Geometry: final body of the model. Coordinates: model frame, mm. Face numbers are marked on the shaded views. Coordinates: 2 decimals unless noted, no trailing zeros. Write each loop counter-clockwise with the first axis right and the second up, starting at its lowest first coordinate (ties: lowest second). Pieces come first, ordered by that corner, then holes.
from build123d import *

# Parameters (mm, degrees)
SKETCH1_W           = 150
SKETCH1_H           = 150
BOSS_EXTRUDE1_DEPTH = 19
SKETCH2_R           = 28
CUT_EXTRUDE1_DEPTH  = 3
SKETCH4_R           = 2.5
CUT_EXTRUDE2_DEPTH  = 6.35


with BuildPart() as part:
    # Sketch1 → Boss-Extrude1 (new body)
    with BuildSketch(Plane(origin=(0, 0, 0), x_dir=(1, 0, 0), z_dir=(0, 1, 0))):
        with Locations((75, 75)):
            Rectangle(SKETCH1_W, SKETCH1_H)
    extrude(amount=BOSS_EXTRUDE1_DEPTH)

    # Sketch2 → Cut-Extrude1 (cut)
    with BuildSketch(Plane(origin=(0, 19, 0), x_dir=(1, 0, 0), z_dir=(0, 1, 0))):
        with Locations((75, 75)):
            Circle(SKETCH2_R)
    extrude(amount=-CUT_EXTRUDE1_DEPTH, mode=Mode.SUBTRACT)

    # Sketch4 → Cut-Extrude2 (cut)
    with BuildSketch(Plane(origin=(0, 19, 0), x_dir=(1, 0, 0), z_dir=(0, 1, 0))):
        with Locations((10, 140)):
            Circle(SKETCH4_R)
        with Locations((140, 140)):
            Circle(SKETCH4_R)
        with Locations((140, 10)):
            Circle(SKETCH4_R)
        with Locations((10, 10)):
            Circle(SKETCH4_R)
    extrude(amount=-CUT_EXTRUDE2_DEPTH, mode=Mode.SUBTRACT)


solid = part.part
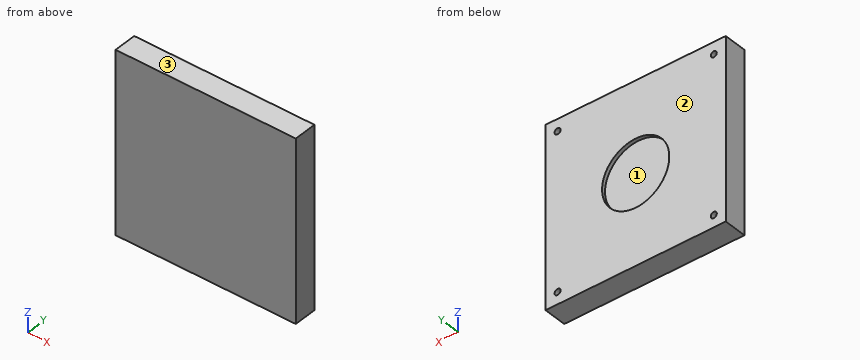
Item 1: Section D-D, the plane x = 10. Output: boundary loops of the cut face in (y, z).
Derived:
outline: (0, -150) - (19, -150) - (19, -142.5) - (12.65, -142.5) - (12.65, -137.5) - (19, -137.5) - (19, -12.5) - (12.65, -12.5) - (12.65, -7.5) - (19, -7.5) - (19, 0) - (0, 0) - close
Item 2: Section C-C, the plane z = -75. Output: boundary loops of the cut face in (x, y), plus the area to 3 significant figures.
Derived:
outline: (0, 0) - (150, 0) - (150, 19) - (103, 19) - (103, 16) - (47, 16) - (47, 19) - (0, 19) - close
area: 2,680 mm2
Item 3: Material intervals for probe 1 along Z at (x, y) = (140, 17.25); probe 2 along X at (y, z) = (14.5, -140); probe 3 along X at (y, z) = (14.25, -138.5), sorted ascending.
Derived:
probe 1: z = -150 to -142.5, -137.5 to -12.5, -7.5 to 0
probe 2: x = 0 to 7.5, 12.5 to 137.5, 142.5 to 150
probe 3: x = 0 to 8, 12 to 138, 142 to 150
Item 4: Section B-B, the plane x = 75. Output: boundary loops of the cut face in (y, z), plus the area to 3 significant figures.
Derived:
outline: (0, -150) - (19, -150) - (19, -103) - (16, -103) - (16, -47) - (19, -47) - (19, 0) - (0, 0) - close
area: 2,680 mm2
Item 5: Pull-direction query (Z, two-part tool) for the marked faces 1, 2 and 3; classes: released by +Z, released by -Z, zero draft, split by the parting line, or undercut.
Derived:
face 1: undercut
face 2: zero draft
face 3: released by +Z
Item 6: Section A-A, the plane z = -10. Output: boundary loops of the cut face in (x, y), plus the area to 3 significant figures.
Derived:
outline: (0, 0) - (150, 0) - (150, 19) - (142.5, 19) - (142.5, 12.65) - (137.5, 12.65) - (137.5, 19) - (12.5, 19) - (12.5, 12.65) - (7.5, 12.65) - (7.5, 19) - (0, 19) - close
area: 2,790 mm2
